Build history of the part. All positions in model axes, mm. A direction names the side the tool comes from. Round coordinates to 2 decimals unless told otherwise and drop trailing zeros. Loops run counter-clockwise (first coordinate to the right, second up) from the corner with the lowest first, then second, coordinate; pieces in that order, holes last. Notation, with made-up numbers: M 9,23 L 62,23 A15 cw 62,30 Z; hole C 82,65.5 d7. An arc over 180 degrees is marked long. One line per item, written item: value.
```python
from build123d import *

# Parameters (mm, degrees)
PAD_DEPTH       = 2.5
SKETCH001_W     = 5
SKETCH001_H     = 10
POCKET_DEPTH    = 5.001
SKETCH002_W     = 10
SKETCH002_H     = 5
POCKET001_DEPTH = 5.001
SKETCH003_W     = 5
SKETCH003_H     = 10
POCKET002_DEPTH = 5.001
SKETCH004_W     = 10
SKETCH004_H     = 5
POCKET003_DEPTH = 5.001
SKETCH005_R     = 2.5
POCKET004_DEPTH = 5.001
SKETCH006_R     = 2.5
POCKET005_DEPTH = 5.001


with BuildPart() as part:
    # Sketch → Pad (new body, symmetric)
    with BuildSketch(Plane.XY):
        Polygon((0, 0), (0, 135), (295, 135), (295, 82.5), (130, 82.5), (130, 0), align=None)
    extrude(amount=PAD_DEPTH, both=True)

    # Sketch001 (on Face8 of Pad) → Pocket (cut, through all)
    with BuildSketch(Plane.XY.offset(2.5)):
        with Locations((292.5, 97.5)):
            Rectangle(SKETCH001_W, SKETCH001_H)
        with Locations((292.5, 117.5)):
            Rectangle(SKETCH001_W, SKETCH001_H)
    extrude(amount=-POCKET_DEPTH, mode=Mode.SUBTRACT)

    # Sketch002 (on Face5 of Pocket) → Pocket001 (cut, through all)
    with BuildSketch(Plane.XY.offset(2.5)):
        with Locations((5, 132.5)):
            Rectangle(SKETCH002_W, SKETCH002_H)
        with Locations((25, 132.5)):
            Rectangle(SKETCH002_W, SKETCH002_H)
        with Locations((45, 132.5)):
            Rectangle(SKETCH002_W, SKETCH002_H)
        with Locations((65, 132.5)):
            Rectangle(SKETCH002_W, SKETCH002_H)
        with Locations((85, 132.5)):
            Rectangle(SKETCH002_W, SKETCH002_H)
        with Locations((105, 132.5)):
            Rectangle(SKETCH002_W, SKETCH002_H)
        with Locations((125, 132.5)):
            Rectangle(SKETCH002_W, SKETCH002_H)
        with Locations((145, 132.5)):
            Rectangle(SKETCH002_W, SKETCH002_H)
        with Locations((165, 132.5)):
            Rectangle(SKETCH002_W, SKETCH002_H)
        with Locations((185, 132.5)):
            Rectangle(SKETCH002_W, SKETCH002_H)
        with Locations((205, 132.5)):
            Rectangle(SKETCH002_W, SKETCH002_H)
        with Locations((225, 132.5)):
            Rectangle(SKETCH002_W, SKETCH002_H)
        with Locations((245, 132.5)):
            Rectangle(SKETCH002_W, SKETCH002_H)
        with Locations((265, 132.5)):
            Rectangle(SKETCH002_W, SKETCH002_H)
        with Locations((285, 132.5)):
            Rectangle(SKETCH002_W, SKETCH002_H)
    extrude(amount=-POCKET001_DEPTH, mode=Mode.SUBTRACT)

    # Sketch003 (on Face4 of Pocket001) → Pocket002 (cut, through all)
    with BuildSketch(Plane.XY.offset(2.5)):
        with Locations((132.5, 95)):
            Rectangle(SKETCH003_W, SKETCH003_H)
        with Locations((132.5, 115)):
            Rectangle(SKETCH003_W, SKETCH003_H)
    extrude(amount=-POCKET002_DEPTH, mode=Mode.SUBTRACT)

    # Sketch004 (on Face4 of Pocket002) → Pocket003 (cut, through all)
    with BuildSketch(Plane.XY.offset(2.5)):
        with Locations((10, 2.5)):
            Rectangle(SKETCH004_W, SKETCH004_H)
        with Locations((30, 2.5)):
            Rectangle(SKETCH004_W, SKETCH004_H)
        with Locations((50, 2.5)):
            Rectangle(SKETCH004_W, SKETCH004_H)
        with Locations((70, 2.5)):
            Rectangle(SKETCH004_W, SKETCH004_H)
        with Locations((90, 2.5)):
            Rectangle(SKETCH004_W, SKETCH004_H)
        with Locations((110, 2.5)):
            Rectangle(SKETCH004_W, SKETCH004_H)
    extrude(amount=-POCKET003_DEPTH, mode=Mode.SUBTRACT)

    # Sketch005 (on Face4 of Pocket003) → Pocket004 (cut, through all)
    with BuildSketch(Plane.XY.offset(2.5)):
        with Locations((20, 110)):
            Circle(SKETCH005_R)
        with Locations((20, 20)):
            Circle(SKETCH005_R)
    extrude(amount=-POCKET004_DEPTH, mode=Mode.SUBTRACT)

    # Sketch006 (on Face4 of Pocket004) → Pocket005 (cut, through all)
    with BuildSketch(Plane.XY.offset(2.5)):
        with Locations((230, 93.2)):
            Circle(SKETCH006_R)
        with Locations((242, 93.2)):
            Circle(SKETCH006_R)
    extrude(amount=-POCKET005_DEPTH, mode=Mode.SUBTRACT)


solid = part.part
```
Item 1: Slice it at B-B, the plane y = 9.5. Give the cut face in (x, z), and give its area (3 significant figures).
Check values:
outline: M 0,-2.5 L 130,-2.5 L 130,2.5 L 0,2.5 Z
area: 650 mm2
Item 2: Drop flat-ended pins along their axis: P1, Ø2.5, axis at x = 245.5, z = 0, coming from the +Y side; P2, Ø1.5, axis at y = 96.5, z = 0.5, coming from the +X side; P3, Ø1.5, axis at y = 2.5, z = -1, coming from the +X side. Give the stop position or say it passes through.
Check values:
P1: stops at y = 130
P2: stops at x = 290
P3: stops at x = 130
Item 3: Wall check: line 1 along X through (y, z) = (114, -0.9); line 2 along X through (y, z) = (109.5, -0.3); line 3 along Y through (x, z) = (242, -1.4). Give the ranges that are in metal, low to high.
Check values:
line 1: x = 0 to 130, 135 to 290
line 2: x = 0 to 17.55, 22.45 to 295
line 3: y = 82.5 to 90.7, 95.7 to 130
Item 4: Which spindle directions (+Z, -Z, +X, -X, +Y, -Y) get a long thin tool onto all of the face, cutting with end or side? Do faces 4 (the face through (45, 2, 0)), 5 (the face through (80, 132, 0)), 6 (the face through (117, 83, -2.5)), 7 (the face through (135, 115, 0)). Say none if no direction does.
Check values:
face 4: +Z, -Z, -Y
face 5: +Z, -Z, +Y
face 6: -Z, +X, -X, +Y, -Y
face 7: +Z, -Z
Item 5: Pull direction Y, two halves, no side cores. Call faces 1 (the face through (185, 130, 0)), 2 (the face through (110, 132, 0)), 3 (the face through (292, 102.5, 0)): pulls with the +Y half, pulls with the -Y half, needs draft (parallel to the pull), parting line crosses it, or undercut.
Check values:
face 1: pulls with the +Y half
face 2: needs draft
face 3: undercut
Item 6: Slice it at A-A, the plane z = -0.05. Give the number of separate pieces and of enclosed holes in the cut face, and give its area (3 significant figures).
Check values:
separate pieces: 1
enclosed holes: 6
area: 24,900 mm2
